from build123d import *

# Parameters (mm, degrees)
F1_DEPTH = 40.259
F3_DEPTH = 25.4
F5_DEPTH = 25.4


with BuildPart() as f1:
    # F0 (on Front) → F1 (new body, symmetric)
    with BuildSketch(Plane.XZ):
        Polygon((0, -0.762), (0, 0), (-37.454836, 63.721383), (-71.236836, 63.721383), (-71.236836, 19.779383), (-46.608452, -14.130657), (-45.846452, -14.130657), (-45.846452, -17.940657), (-46.608452, -17.940657), (-64.46274, -56.418067), (-64.46274, -101.376067), (-17.47274, -101.376067), (4.734051, -50.098072), (4.734051, -49.336072), (8.544051, -49.336072), (8.544051, -50.098072), (33.19607, -101.376067), (80.69407, -101.376067), (80.69407, -48.036067), (63.988247, -23.151609), (63.226247, -23.151609), (63.226247, -19.341609), (63.988247, -19.341609), (80.262104, 7.029165), (80.262104, 60.877165), (47.496104, 60.877165), (3.81, 0), (3.81, -0.762), align=None)
    extrude(amount=F1_DEPTH, both=True)

    # F2 (on face) → F3 (cut)
    with BuildSketch(Plane.XZ.offset(40.259)):
        with BuildLine():
            ThreePointArc((-52.245846, 16.276482), (-38.390892, 13.469409), (-30.523199, 25.214145))
            ThreePointArc((-30.523199, 25.214145), (-30.687283, 27.249046), (-31.175296, 29.231365))
            ThreePointArc((-31.175296, 29.231365), (-49.874912, 36.032865), (-52.245846, 16.276482))
        make_face()
        with BuildLine():
            ThreePointArc((-31.175296, 29.231365), (-30.687283, 27.249046), (-30.523199, 25.214145))
            ThreePointArc((-30.523199, 25.214145), (-38.390892, 13.469409), (-52.245846, 16.276482))
            Line((-52.245846, 16.276482), (-37.573051, -6.265247))
            ThreePointArc((-37.573051, -6.265247), (-34.402313, -16.422015), (-36.996162, -26.741195))
            Line((-36.996162, -26.741195), (-50.912392, -56.731777))
            ThreePointArc((-50.912392, -56.731777), (-28.804068, -48.448298), (-14.646231, -67.34141))
            ThreePointArc((-14.646231, -67.34141), (-14.651472, -67.795631), (-14.667193, -68.249609))
            Line((-14.667193, -68.249609), (-3.134057, -43.394785))
            ThreePointArc((-3.134057, -43.394785), (7.514222, -40.45337), (17.917042, -44.17078))
            Line((17.917042, -44.17078), (32.565061, -74.639729))
            ThreePointArc((32.565061, -74.639729), (41.062727, -50.578546), (66.172654, -55.121942))
            Line((66.172654, -55.121942), (50.676871, -30.211112))
            ThreePointArc((50.676871, -30.211112), (47.597224, -20.692297), (49.331598, -10.839176))
            Line((49.331598, -10.839176), (65.190411, 14.949097))
            ThreePointArc((65.190411, 14.949097), (49.396243, 10.062519), (42.155779, 24.925563))
            Line((42.155779, 24.925563), (13.816384, -10.301067))
            ThreePointArc((13.816384, -10.301067), (0.898878, -16.153519), (-11.474751, -9.224849))
            Line((-11.474751, -9.224849), (-31.175296, 29.231365))
        make_face()
        with BuildLine():
            ThreePointArc((67.143639, 21.716436), (56.06138, 34.31298), (42.155779, 24.925563))
            ThreePointArc((42.155779, 24.925563), (49.396243, 10.062519), (65.190411, 14.949097))
            Line((65.190411, 14.949097), (65.331844, 15.179083))
            ThreePointArc((65.331844, 15.179083), (66.682311, 18.324549), (67.143639, 21.716436))
        make_face()
        with BuildLine():
            Line((-53.138839, -61.529947), (-50.912392, -56.731777))
            ThreePointArc((-50.912392, -56.731777), (-52.187514, -59.055738), (-53.138839, -61.529947))
        make_face()
        with BuildLine():
            ThreePointArc((-14.646231, -67.34141), (-28.804068, -48.448298), (-50.912392, -56.731777))
            Line((-50.912392, -56.731777), (-53.138839, -61.529947))
            ThreePointArc((-53.138839, -61.529947), (-37.718241, -86.732836), (-14.667193, -68.249609))
            ThreePointArc((-14.667193, -68.249609), (-14.651472, -67.795631), (-14.646231, -67.34141))
        make_face()
        with BuildLine():
            Line((65.331844, 15.179083), (65.190411, 14.949097))
            ThreePointArc((65.190411, 14.949097), (65.261739, 15.063714), (65.331844, 15.179083))
        make_face()
        with BuildLine():
            Line((68.871818, -59.461086), (66.172654, -55.121942))
            ThreePointArc((66.172654, -55.121942), (41.062727, -50.578546), (32.565061, -74.639729))
            ThreePointArc((32.565061, -74.639729), (54.527629, -86.95802), (70.633667, -67.601103))
            ThreePointArc((70.633667, -67.601103), (70.188163, -63.43685), (68.871818, -59.461086))
        make_face()
        with BuildLine():
            ThreePointArc((68.871818, -59.461086), (67.663637, -57.203555), (66.172654, -55.121942))
            Line((66.172654, -55.121942), (68.871818, -59.461086))
        make_face()
    extrude(amount=-F3_DEPTH, mode=Mode.SUBTRACT)

    # F4 (on face) → F5 (cut)
    with BuildSketch(Plane(origin=(0, 40.259, 0), x_dir=(-1, 0, 0), z_dir=(0, 1, 0))):
        with BuildLine():
            ThreePointArc((-65.726989, 18.3497), (-51.872034, 15.542628), (-44.004341, 27.287363))
            ThreePointArc((-44.004341, 27.287363), (-44.168425, 29.322264), (-44.656439, 31.304583))
            ThreePointArc((-44.656439, 31.304583), (-63.356054, 38.106083), (-65.726989, 18.3497))
        make_face()
        with BuildLine():
            ThreePointArc((-44.656439, 31.304583), (-44.168425, 29.322264), (-44.004341, 27.287363))
            ThreePointArc((-44.004341, 27.287363), (-51.872034, 15.542628), (-65.726989, 18.3497))
            Line((-65.726989, 18.3497), (-51.054193, -4.192029))
            ThreePointArc((-51.054193, -4.192029), (-46.106839, -17.471409), (-49.249755, -31.289525))
            Line((-49.249755, -31.289525), (-65.967989, -60.914299))
            ThreePointArc((-65.967989, -60.914299), (-43.823018, -51.54992), (-29.139468, -70.588952))
            ThreePointArc((-29.139468, -70.588952), (-29.144731, -71.044099), (-29.160516, -71.499002))
            Line((-29.160516, -71.499002), (-15.92485, -43.967853))
            ThreePointArc((-15.92485, -43.967853), (-5.553349, -41.629648), (4.695866, -44.456098))
            Line((4.695866, -44.456098), (19.922124, -74.438221))
            ThreePointArc((19.922124, -74.438221), (26.714122, -49.040464), (52.697492, -53.045686))
            Line((52.697492, -53.045686), (37.20171, -28.134856))
            ThreePointArc((37.20171, -28.134856), (34.122063, -18.616042), (35.856437, -8.762921))
            Line((35.856437, -8.762921), (52.887628, 18.931776))
            ThreePointArc((52.887628, 18.931776), (37.702376, 15.634645), (30.692658, 29.502839))
            Line((30.692658, 29.502839), (9.262503, -6.26221))
            ThreePointArc((9.262503, -6.26221), (-3.243304, -11.839034), (-15.496504, -5.727138))
            Line((-15.496504, -5.727138), (-44.656439, 31.304583))
        make_face()
        with BuildLine():
            ThreePointArc((55.863387, 27.100566), (44.369981, 39.743119), (30.692658, 29.502839))
            ThreePointArc((30.692658, 29.502839), (37.702376, 15.634645), (52.887628, 18.931776))
            Line((52.887628, 18.931776), (54.840929, 22.10807))
            ThreePointArc((54.840929, 22.10807), (55.605147, 24.552506), (55.863387, 27.100566))
        make_face()
        with BuildLine():
            ThreePointArc((-29.139468, -70.588952), (-43.823018, -51.54992), (-65.967989, -60.914299))
            ThreePointArc((-65.967989, -60.914299), (-54.264793, -89.507252), (-29.160516, -71.499002))
            ThreePointArc((-29.160516, -71.499002), (-29.144731, -71.044099), (-29.139468, -70.588952))
        make_face()
        with BuildLine():
            Line((54.840929, 22.10807), (52.887628, 18.931776))
            ThreePointArc((52.887628, 18.931776), (53.981487, 20.447844), (54.840929, 22.10807))
        make_face()
        with BuildLine():
            Line((55.396657, -57.38483), (52.697492, -53.045686))
            ThreePointArc((52.697492, -53.045686), (26.714122, -49.040464), (19.922124, -74.438221))
            ThreePointArc((19.922124, -74.438221), (42.056096, -84.669013), (57.158505, -65.524847))
            ThreePointArc((57.158505, -65.524847), (56.713002, -61.360595), (55.396657, -57.38483))
        make_face()
        with BuildLine():
            ThreePointArc((55.396657, -57.38483), (54.188476, -55.1273), (52.697492, -53.045686))
            Line((52.697492, -53.045686), (55.396657, -57.38483))
        make_face()
    extrude(amount=-F5_DEPTH, mode=Mode.SUBTRACT)


solid = f1.part
Verification items for the finished model (mm, model axes). A direction names the side the tool comes from. Give positions to 0.01 mm unless a question says otherwise; leave off trailing zeros. Loops run counter-clockwise (first coordinate to the right, second up) from the corner with the lowest first, then second, coordinate; pieces in that order, holes last. Notation, with made-up numbers: (37, 55.25) - (65, 55.25) arc R23 ccw to (65, 86.25) - close; hole circle Ø4 at (-21, 23). An arc over 180 degrees is marked (long way). Write item = value, one per line. Start each with the question number.
Q1. Tool access check on faces 1 (the face through (-6.525, -0.564, -76.096)), 2 (the face through (-55.41, -0.56, -36.91)), 3 (the face through (28.184, -27.737, 7.559)), 4 (the face through (-18.465, -0.564, 31.415)), 5 (the face through (-34.132, 27.737, -18.757)). Record the directions out of +Z, -Z, +X, -X, +Y, -Y that give a thin tool (end or side, any length) a straight path to the whole face; none if there is none.
Q2. Depth check by flat-ended pin: P1, Ø4, axis at y = 24, z = 7.5, coming from the -X side; P2, Ø3, axis at x = 2, y = 10.5, coming from the +Z side; P3, Ø6, axis at x = 19.5, y = 10.5, coming from the +Z side; P4, Ø6, axis at x = 31, y = 16, coming from the -Z side. Enter the tip coordinate at first touch or a pass-through.
Q3. Cross-section at D-D, the plane z = 42. Enter the section's corners in (x, y), and give its area (3 significant figures).
Q4. Cross-section at C-C, the plane x = -43.5. Enter the section's corners in (y, z), and give its area (3 significant figures).
Q5. Cross-section at A-A, the plane z = 4. Enter the section's corners in (x, y).
Q6. Mould release check, pull along X, two halves, no side actions. Record for faces 6 (the face through (57, -1, -101.376)), 7 (the face through (2, -1, -0.762)), 8 (the face through (80.694, -1, -75)), 9 (the face through (25.139, -27.737, -59.192)): released by +X, released by -X, zero draft, split by the parting line, or undercut.
Q7. Thickness scan on line 1 (X direction, y = -29, z = -77); line 2 (X direction, y = 27.5, z = -62); line 3 (Z direction, x = 51.5, y = 19.5). Record the ranges inside material, lowest first.
Q8. Cross-section at B-B, the plane y = -11. Enter the section's corners in (x, z), and give its area (3 significant figures).
Answer key:
q1.face_1 = -Z, +Y, -Y
q1.face_2 = -X, +Y, -Y
q1.face_3 = -Y
q1.face_4 = +Z, +Y, -Y
q1.face_5 = +Y
q2.P1 = -63.77
q2.P2 = -0.76
q2.P3 = 26.04
q2.P4 = -101.38
q3.outline = (-71.24, -40.26) - (-24.69, -40.26) - (-24.69, 40.26) - (-71.24, 40.26) - close; (33.95, -40.26) - (80.26, -40.26) - (80.26, 40.26) - (33.95, 40.26) - close
q3.area = 7,480 mm^2
q4.outline = (-40.26, -101.38) - (40.26, -101.38) - (40.26, -84.26) - (14.86, -84.26) - (14.86, -38.26) - (40.26, -38.26) - (40.26, 3.67) - (14.86, 3.67) - (14.86, 39.8) - (40.26, 39.8) - (40.26, 63.72) - (-40.26, 63.72) - (-40.26, 37.91) - (-14.86, 37.91) - (-14.86, 2.84) - (-40.26, 2.84) - (-40.26, -40.76) - (-14.86, -40.76) - (-14.86, -84.76) - (-40.26, -84.76) - close
q4.area = 9,200 mm^2
q5.outline = (-59.78, -40.26) - (-44.25, -40.26) - (-44.25, -14.86) - (-18.25, -14.86) - (-18.25, -40.26) - (-2.35, -40.26) - (-2.35, 40.26) - (-15.41, 40.26) - (-15.41, 14.86) - (-43.71, 14.86) - (-43.71, 40.26) - (-59.78, 40.26) - close; (6.68, -40.26) - (25.32, -40.26) - (25.32, -14.86) - (58.46, -14.86) - (58.46, -40.26) - (78.39, -40.26) - (78.39, 40.26) - (56.39, 40.26) - (56.39, 14.86) - (23.16, 14.86) - (23.16, 40.26) - (6.68, 40.26) - close
q6.face_6 = zero draft
q6.face_7 = undercut
q6.face_8 = released by +X
q6.face_9 = undercut
q7.line_1 = -64.46 to -51.48, -17.18 to -6.92, 21.48 to 33.65, 68.24 to 80.69
q7.line_2 = -64.46 to -56.84, -13.61 to -0.42, 14.27 to 24.59, 66.54 to 80.69
q7.line_3 = -101.38 to -90.09, -35.28 to -3.51, 38.87 to 60.88
q8.outline = (-71.24, 19.78) - (-46.61, -14.13) - (-45.85, -14.13) - (-45.85, -17.94) - (-46.61, -17.94) - (-64.46, -56.42) - (-64.46, -101.38) - (-17.47, -101.38) - (4.73, -50.1) - (4.73, -49.34) - (8.54, -49.34) - (8.54, -50.1) - (33.2, -101.38) - (80.69, -101.38) - (80.69, -48.04) - (63.99, -23.15) - (63.23, -23.15) - (63.23, -19.34) - (63.99, -19.34) - (80.26, 7.03) - (80.26, 60.88) - (47.5, 60.88) - (3.81, 0) - (3.81, -0.76) - (0, -0.76) - (0, 0) - (-37.45, 63.72) - (-71.24, 63.72) - close
q8.area = 18,700 mm^2
